Drawing for the job (mm, zero at the part's lowest x, y, z). Round coordinates to 2 decimals unless told otherwise and drop trailing zeros. Write each loop counter-clockwise with the first axis right and the second up, starting at its lowest first coordinate (ties: lowest second). Pieces come first, ordered by that corner, then holes. Notation, with made-up numbers: M 1.25,33 L 60.25,33 A23 cw 60.25,58 Z; hole C 85.5,48 d4. An arc over 180 degrees is marked long. Use a Markdown table: item, result. Add a question column.
1) Slice it at A-A on z = 6.35. Write the cut outline in (x, y).
2) Drop a flat-ended pin along its axis: P1, Ø3, axis at y = 3, z = 6.5, coming from the -X side. Give the stop position or say it passes through.
3) Slice it at C-C on y = 1. Write the cut outline in (x, z) (1 decimal).
4) Two-plate mould, pull along Z, no slides. Class the marked faces 1, 2 and 3: released by +Z, released by -Z, zero draft, split by the parting line, or undercut.
5) Wall check: probe 1 along Y at (x, z) = (8.1, 6.35); probe 2 along Z at (x, y) = (5.75, 3.5) (1 decimal); probe 3 along X at (y, z) = (6, 4). Give the ranges that are in metal, low to high.
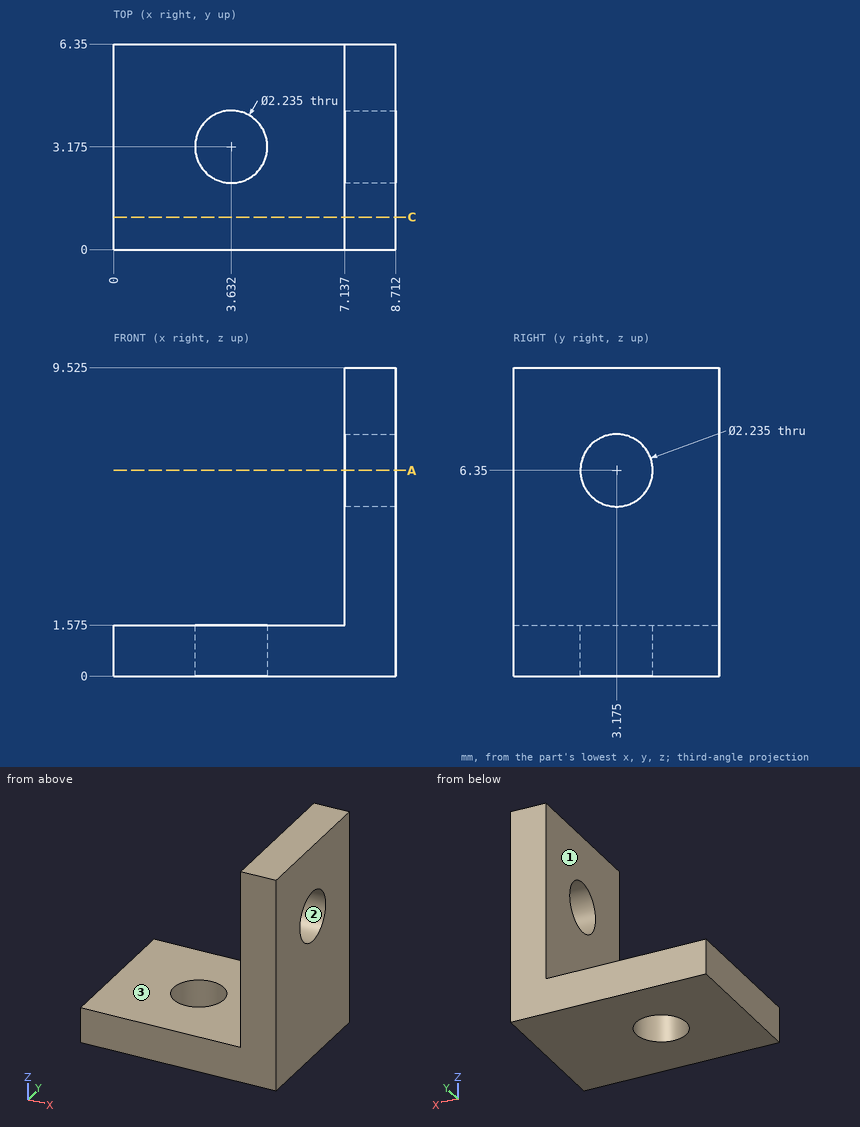
Entries:
| question | item | result |
|---|---|---|
| 1 | outline | M 7.14,0 L 8.71,0 L 8.71,2.06 L 7.14,2.06 Z; M 7.14,4.29 L 8.71,4.29 L 8.71,6.35 L 7.14,6.35 Z |
| 2 | P1 | stops at x = 7.14 |
| 3 | outline | M 0,0 L 8.7,0 L 8.7,9.5 L 7.1,9.5 L 7.1,1.6 L 0,1.6 Z |
| 4 | face 1 | zero draft |
| 4 | face 2 | undercut |
| 4 | face 3 | released by +Z |
| 5 | probe 1 | y = 0 to 2.06, 4.29 to 6.35 |
| 5 | probe 2 | z = 0 to 1.6 |
| 5 | probe 3 | x = 7.14 to 8.71 |
